Design review of the part built by this model. Coordinates are the model's own, in mm. A direction names the side the tool comes from. Give positions to 0.01 mm unless a question says otherwise; leave off trailing zeros. Write each loop counter-clockwise with the first axis right and the second up, starting at its lowest first coordinate (ties: lowest second). Pieces come first, ordered by that corner, then holes. Notation, with made-up numbers: (78, 39.5) -> (88, 39.5) arc R9 ccw to (88, 49.5) -> close; hole circle Ø3 at (-5, 76). An arc over 180 degrees is marked (long way). Write each question's results on one line, items separated by ' | '. Start each with the question number.
(1) Mouldability with a two-part tool opening along Y and no side actions: class faces 1 (the face through (5.07, -32.217, -36.774)), 2 (the face through (53, -29, 30)), 3 (the face through (10, 31, 35)) as released by +Y, released by -Y, zero draft, split by the parting line, or undercut.
(2) To check wall thickness, follow probe 1 along Y at (x, z) = (2, -35); probe 2 along Z at (x, y) = (53.5, -37); probe 3 along X at (y, z) = (27, 28.5). State the ranges of each line that lie inside material, in increasing order.
(3) Clearance check with flat-ended pins moving along their axes: pin 1 (2.5 mm diameter, centred on x = 39, z = -36, fed in from +Y); pin 2 (2 mm diameter, centred on x = 69, y = -30, fed in from -Z); pin 3 (2.5 mm diameter, centred on x = 70, y = -36.5, fed in from +Z); pin 4 (6 mm diameter, centred on y = -29.5, z = -33.5, fed in from +X). State where each tip first meets the part, or that it passes through.
(4) For faces 4 (the face through (54, -28, -36)), 5 (the face through (0, 1, 38)), 6 (the face through (10, -33, 38)), 7 (the face through (53, 42, -26)), 8 (the face through (53, 30, 29)), list the 3-axis set-ups (+Z, -Z, +X, -X, +Y, -Y) from which the entire face can be reached by the end or side of a thin tool; tool diameter is ignored.
(5) Take a section at A-A (y = 35). State the section outline as (x, z) points.
(6) Take a section at D-D (y = 0). State the section outline as (x, z) points.
(7) Take a section at B-B (x = 75). State the section outline as (y, z) points.
from build123d import *

# Parameters (mm, degrees)
BOSS_EXTRUDE1_DEPTH  = 97.5
SKETCH2_R            = 36.5
BOSS_EXTRUDE2_DEPTH  = 1.6
BOSS_EXTRUDE4_START  = -1.6
SKETCH3_R            = 7
BOSS_EXTRUDE4_DEPTH  = 34
CUT_EXTRUDE1_START   = -24.820064241
CUT_EXTRUDE1_DEPTH   = 24.820064241
SKETCH12_OUTSIDE_W   = 123.824
SKETCH12_OUTSIDE_H   = 123.824
CUT_EXTRUDE2_DEPTH   = 87.5
M6_CLEARANCE_HOLE2_D = 6.6
FILLET1_R            = 5
CHAMFER1_SIZE        = 1


with BuildPart() as part:
    # Sketch1 → Boss-Extrude1 (new body)
    with BuildSketch(Plane(origin=(0, 0, 0), x_dir=(0, 0, -1), z_dir=(1, 0, 0))):
        with BuildLine():
            Line((-31, 43), (31, 43))
            ThreePointArc((31, 43), (39.485281374, 39.485281374), (43, 31))
            Line((43, 31), (43, -31))
            ThreePointArc((43, -31), (39.485281374, -39.485281374), (31, -43))
            Line((31, -43), (-31, -43))
            ThreePointArc((-31, -43), (-39.485281374, -39.485281374), (-43, -31))
            Line((-43, -31), (-43, 31))
            ThreePointArc((-43, 31), (-39.485281374, 39.485281374), (-31, 43))
        make_face()
    extrude(amount=BOSS_EXTRUDE1_DEPTH)

    # Sketch2 → Boss-Extrude2 (add)
    with BuildSketch(Plane.ZY):
        Circle(SKETCH2_R)
    extrude(amount=BOSS_EXTRUDE2_DEPTH)

    # Sketch3 → Boss-Extrude4 (add)
    with BuildSketch(Plane.ZY.offset(1.6).offset(BOSS_EXTRUDE4_START)):
        with Locations(Location((0, 0, 0), (0, 0, 180))):
            Circle(SKETCH3_R)
    extrude(amount=BOSS_EXTRUDE4_DEPTH)

    # Sketch4 → Cut-Extrude1 (cut)
    with BuildSketch(Plane.ZY.offset(34).offset(CUT_EXTRUDE1_START)):
        with BuildLine():
            Line((-4.898979486, 5), (4.898979486, 5))
            ThreePointArc((4.898979486, 5), (0, 7), (-4.898979486, 5))
        make_face()
    extrude(amount=CUT_EXTRUDE1_DEPTH, mode=Mode.SUBTRACT)

    # Sketch12 outside → Cut-Extrude2 (cut)
    with BuildSketch(Plane(origin=(97.5, 0, 0), x_dir=(0, 0, -1), z_dir=(1, 0, 0))):
        Rectangle(SKETCH12_OUTSIDE_W, SKETCH12_OUTSIDE_H)
        Polygon((-28, 43), (28, 43), (28, 28), (43, 28), (43, -28), (28, -28), (28, -43), (-28, -43), (-28, -28), (-43, -28), (-43, 28), (-28, 28), align=None, mode=Mode.SUBTRACT)
    extrude(amount=-CUT_EXTRUDE2_DEPTH, mode=Mode.SUBTRACT)

    # M6 Clearance Hole2 (through all)
    with Locations(Plane.ZY):
        with Locations((-35, 35), (35, 35), (35, -35), (-35, -35)):
            Hole(M6_CLEARANCE_HOLE2_D / 2)

    # Fillet1
    fillet1_edges = [part.edges().sort_by_distance(p)[0] for p in [
        (53.75, 28, 28),
        (53.75, 28, 43),
        (53.75, -28, 43),
        (53.75, -28, 28),
        (53.75, -43, 28),
        (53.75, -43, -28),
        (53.75, -28, -28),
        (53.75, -28, -43),
        (53.75, 28, -43),
        (53.75, 28, -28),
        (53.75, 43, -28),
        (53.75, 43, 28),
    ]]
    fillet(fillet1_edges, radius=FILLET1_R)

    # Chamfer1
    chamfer1_edges = [part.edges().sort_by_distance(p)[0] for p in [
        (-34, -6.453404388, 2.711747002),
    ]]
    chamfer(chamfer1_edges, length=CHAMFER1_SIZE)


solid = part.part
Report:
1) face 1: undercut | face 2: released by -Y | face 3: zero draft
2) probe 1: -42.31 to -38.3, -31.7 to 31.7, 38.3 to 42.31 | probe 2: -28 to 28 | probe 3: 0 to 97.5
3) pin 1: y = 28 | pin 2: z = -30 | pin 3: z = 28 | pin 4: x = 97.5
4) face 4: -Z, +X, -Y | face 5: -X | face 6: +Z, +X, -Y | face 7: -Z, +X, +Y | face 8: +Z, +X, +Y
5) outline: (-1.6, -10.36) -> (0, -10.36) -> (0, -31.7) -> (10, -31.7) -> (10, -28) -> (97.5, -28) -> (97.5, 28) -> (10, 28) -> (10, 31.7) -> (0, 31.7) -> (0, 10.36) -> (-1.6, 10.36) -> close; (0, -42.31) -> (10, -42.31) -> (10, -38.3) -> (0, -38.3) -> close; (0, 38.3) -> (10, 38.3) -> (10, 42.31) -> (0, 42.31) -> close
6) outline: (-34, -6) -> (-33, -7) -> (-1.6, -7) -> (-1.6, -36.5) -> (0, -36.5) -> (0, -43) -> (97.5, -43) -> (97.5, 43) -> (0, 43) -> (0, 36.5) -> (-1.6, 36.5) -> (-1.6, 7) -> (-33, 7) -> (-34, 6) -> close
7) outline: (-43, -23) arc R5 ccw to (-38, -28) -> (-33, -28) arc R5 cw to (-28, -33) -> (-28, -38) arc R5 ccw to (-23, -43) -> (23, -43) arc R5 ccw to (28, -38) -> (28, -33) arc R5 cw to (33, -28) -> (38, -28) arc R5 ccw to (43, -23) -> (43, 23) arc R5 ccw to (38, 28) -> (33, 28) arc R5 cw to (28, 33) -> (28, 38) arc R5 ccw to (23, 43) -> (-23, 43) arc R5 ccw to (-28, 38) -> (-28, 33) arc R5 cw to (-33, 28) -> (-38, 28) arc R5 ccw to (-43, 23) -> close
